```python
from build123d import *

# Parameters (mm, degrees)
SKETCH1_R           = 3
BOSS_EXTRUDE1_DEPTH = 4
FILLET1_R           = 4


with BuildPart() as part:
    # Sketch1 → Boss-Extrude1 (new body)
    with BuildSketch(Plane(origin=(0, 0, 0), x_dir=(1, 0, 0), z_dir=(0, 1, 0))):
        with BuildLine():
            Line((-8, 0), (-8, 16))
            Line((-8, 16), (8, 16))
            Line((8, 16), (8, 0))
            ThreePointArc((8, 0), (0, -8), (-8, 0))
        make_face()
        with Locations(Location((0, 0, 0), (0, 0, 270))):
            Circle(SKETCH1_R, mode=Mode.SUBTRACT)
    extrude(amount=BOSS_EXTRUDE1_DEPTH)

    # Fillet1
    fillet1_edges = [part.edges().sort_by_distance(p)[0] for p in [
        (-8, 2, -16),
        (8, 2, -16),
    ]]
    fillet(fillet1_edges, radius=FILLET1_R)


solid = part.part
```
For this review, take the finished solid that the model builds, in its own axes (mm). Coordinates: 2 decimals unless noted, no trailing zeros. Order: outer loops, then holes, each group sorted by start corner. A loop starts at its lowest first (then second) coordinate and runs counter-clockwise, first axis right, second up. Notation, with made-up numbers: (26.25, 19.5) -> (76.25, 19.5) arc R6 cw to (76.25, 23.5) -> close; hole circle Ø3 at (-19.5, 18). An arc over 180 degrees is marked (long way). Use CSV: the item, a comma, the result in double quotes. Start each with the question number.
Item 1: We need section B-B, the plane y = 3.25. Give the boundary of the cut face in (x, z).
Item 2: We need section D-D, the plane x = -3.5. Give the boundary of the cut face in (y, z).
Item 3: We need section C-C, the plane z = 1.25. Give the boundary of the cut face in (x, y).
Item 4: We need section A-A, the plane x = 0. Give the boundary of the cut face in (y, z).
Item 5: Wall thickness on probe 1 along X at (y, z) = (2.6, 1.25); probe 2 along Z at (x, y) = (0.25, 2); probe 3 along X at (y, z) = (2.75, -2.75): over which ranges is each line inside the solid? List them lowest first.
Derived:
1,outline,"(-8, -12) arc R4 ccw to (-4, -16) -> (4, -16) arc R4 ccw to (8, -12) -> (8, 0) arc R8 ccw to (-8, 0) -> close; hole circle Ø6 at (0, 0)"
2,outline,"(0, -16) -> (4, -16) -> (4, 7.19) -> (0, 7.19) -> close"
3,outline,"(-7.9, 0) -> (-2.73, 0) -> (-2.73, 4) -> (-7.9, 4) -> close; (2.73, 0) -> (7.9, 0) -> (7.9, 4) -> (2.73, 4) -> close"
4,outline,"(0, -16) -> (4, -16) -> (4, -3) -> (0, -3) -> close; (0, 3) -> (4, 3) -> (4, 8) -> (0, 8) -> close"
5,probe 1,"x = -7.9 to -2.73, 2.73 to 7.9"
5,probe 2,"z = -16 to -2.99, 2.99 to 8"
5,probe 3,"x = -8 to -1.2, 1.2 to 8"
